Source: three-view drawing plus pictorial views. Frame: mm from the lowest corner of the part. A direction names the side the tool comes from. Round coordinates to 2 decimals unless told otherwise and drop trailing zeros. Order: outer loops, then holes, each group sorted by start corner. A loop starts at its lowest first (then second) coordinate and runs counter-clockwise, first axis right, second up. Notation, with made-up numbers: (-12.75, -26) -> (1.25, -26) arc R22 cw to (1.25, 1) -> close; hole circle Ø5 at (7.5, 32.25). An arc over 180 degrees is marked (long way). Answer as CSV lines item,"result". Start each with the question number.
1) Access query for the marked faces 4, 5 and 6. Directions: +Z, -Z, +X, -X, +Y, -Y. A direction counts if a zero-diameter tool reaches every point of the face in a straight line with its end or side. Return the directions, or none.
2) Mould query, pull axis Z, two halves, no side actions, for the marked faces 1, 2 and 3. Classes: +Z half, -Z half, draft (parallel to the pull), parting line (faces both ways), or undercut.
3) Section query A-A, the plane y = 1. Output: boundary loops of the cut face in (x, z).
4) Section query C-C, the plane z = 2.5. Output: boundary loops of the cut face in (x, y) (1 decimal).
5) First-contact query: P1, Ø3, axis at x = 4.5, z = 6, coming from the +Y side; P2, Ø1.7, axis at y = 1, z = 3, coming from the -X side. Flat tips, straight axial feed; report the tip coordinate or a pass-through.
6) Line query: L1, parallel to X at y = 1.5, z = 9.75; L2, parallel to Y at x = 1, z = 1; L3, parallel to Y at x = 6, z = 7 (1 decimal). Output: solid intervals per line, ascending.
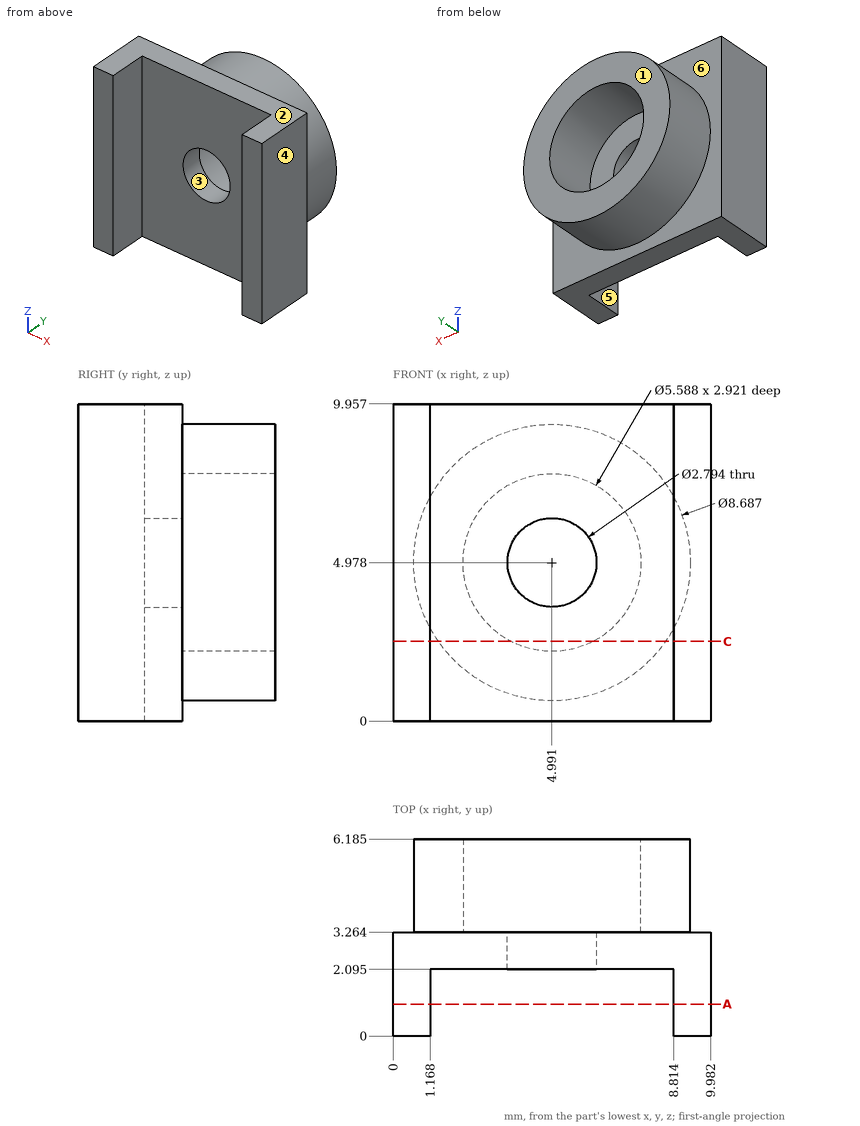
Findings:
1,face 4,"+Z, -Z, +X, +Y, -Y"
1,face 5,"+Z, -Z, -Y"
1,face 6,"+Y"
2,face 1,"draft"
2,face 2,"+Z half"
2,face 3,"undercut"
3,outline,"(0, 0) -> (1.17, 0) -> (1.17, 9.96) -> (0, 9.96) -> close; (8.81, 0) -> (9.98, 0) -> (9.98, 9.96) -> (8.81, 9.96) -> close"
4,outline,"(0, 0) -> (1.2, 0) -> (1.2, 2.1) -> (8.8, 2.1) -> (8.8, 0) -> (10, 0) -> (10, 3.3) -> (8.6, 3.3) -> (8.6, 6.2) -> (6.3, 6.2) -> (6.3, 3.3) -> (3.7, 3.3) -> (3.7, 6.2) -> (1.4, 6.2) -> (1.4, 3.3) -> (0, 3.3) -> close"
5,P1,"stops at y = 3.26"
5,P2,"stops at x = 0"
6,L1,"x = 0 to 1.17, 8.81 to 9.98"
6,L2,"y = 0 to 3.26"
6,L3,"y = 2.1 to 3.3"
